For this review, take the finished solid that the model builds, in its own axes (mm). A direction names the side the tool comes from. Give positions to 0.01 mm unless a question says otherwise; leave off trailing zeros. Write each loop counter-clockwise with the first axis right and the second up, starting at its lowest first coordinate (ties: lowest second). Pieces come first, ordered by that corner, then holes.
Q1. We need section A-A (x = -74). Write out the cut boundary in (y, z), then the cut area to 3 significant figures.
Q2. We need section B-B (z = 41). Write out the cut boundary in (x, y), then the cut area to 3 significant figures.
Q3. Insertion check: P1, Ø1, axis at x = 100.5, z = 60, coming from the -Y side; P2, Ø1.4, axis at x = 12.5, y = 40.5, coming from the -Z side; P3, Ø5, axis at x = 157, z = 21.5, coming from the +Y side; P4, Ø5, axis at x = 86.5, y = 39, coming from the -Z side. Each pin has a flat end and moves straight along its axis. Give the tip position at first contact, or say it passes through.
Q4. Mouldability with a two-part tool opening along Y and no side actions: class faces 1 (the flat face through (2, 76, 10)), 2 (the flat face through (19.509, 47, 4)), 3 (the flat face through (4, 89.566, 7)), 4 (the cylindrical face through (4.839, 69.563, 4.056)) as released by +Y, released by -Y, zero draft, split by the parting line, or undercut.
Q5. For line 1 (X direction, y = 81.5, z = 18); line 2 (Z direction, x = 79, y = 84.5); line 3 (X direction, y = 51, z = 5.5), list the stretches that pass through material, from the lowest coordinate up.
Q6. We need section D-D (z = 20). Write out the cut boundary in (x, y).
Q7. We need section C-C (x = 161). Write out the cut boundary in (y, z).
Q8. Machinability: for faces 5 (the flat face through (-17.852, 25, 5)), 6 (the flat face through (-10.491, 47, 4)), 7 (the flat face through (4, 27, 10)), 8 (the flat face through (2, 74, 70)), 9 (the flat face through (26.87, 25, 5)), which of the approach directions +Z, -Z, +X, -X, +Y, -Y give a long, thin tool a straight path to every point of the face, cutting with its end or side? Answer none if there is none.
```python
from build123d import *

# Parameters (mm, degrees)
ESQUISSE2_W              = 430
ESQUISSE2_H              = 60
BOSS_EXTRU_1_DEPTH       = 80
ESQUISSE3_W              = 410
ESQUISSE3_H              = 60
ENL_V_MAT_EXTRU_2_DEPTH  = 50
BOSS_EXTRU_3_DEPTH       = 60
BOSS_EXTRU_4_DEPTH       = 20
ESQUISSE12_W             = 37.299463168
ESQUISSE12_H             = 2.901511437
ENL_V_MAT_EXTRU_3_DEPTH  = 80
ESQUISSE14_W             = 217.702790891
ESQUISSE14_H             = 66.731599488
ENL_V_MAT_EXTRU_4_DEPTH  = 80
ESQUISSE16_W             = 132.026208669
ESQUISSE16_H             = 23.789258621
ENL_V_MAT_EXTRU_5_DEPTH  = 80
ESQUISSE17_W             = 231.982221262
ESQUISSE17_H             = 63.124798286
ENL_V_MAT_EXTRU_6_DEPTH  = 80
ESQUISSE18_R             = 15
ENL_V_MAT_EXTRU_7_DEPTH  = 80
ENL_V_MAT_EXTRU_8_DEPTH  = 10
CONG_3_R                 = 2
CONG_4_R                 = 2
ESQUISSE26_W             = 44.72135955
ESQUISSE26_H             = 10
BOSS_EXTRU_5_DEPTH       = 10
ENL_V_MAT_EXTRU_9_DEPTH  = 10
ESQUISSE27_R             = 2
ENL_V_MAT_EXTRU_11_DEPTH = 10


with BuildPart() as part:
    # Esquisse2 → Boss.-Extru.1 (new body)
    with BuildSketch(Plane.XY):
        with Locations((4.509056244, 59.566253575)):
            Rectangle(ESQUISSE2_W, ESQUISSE2_H)
    extrude(amount=BOSS_EXTRU_1_DEPTH)

    # Esquisse3 → Enlèv. mat.-Extru.2 (cut)
    with BuildSketch(Plane(origin=(0, 89.566253575, 0), x_dir=(1, 0, 0), z_dir=(0, 1, 0))):
        with Locations((4.509056244, -40)):
            Rectangle(ESQUISSE3_W, ESQUISSE3_H)
    extrude(amount=-ENL_V_MAT_EXTRU_2_DEPTH, mode=Mode.SUBTRACT)

    # Esquisse5 → Boss.-Extru.3 (add)
    with BuildSketch(Plane.XY.offset(10)):
        Polygon((-200.490943756, 59.566253575), (-200.490943756, 39.566253575), (4.509056244, 39.566253575), align=None)
        Polygon((209.509056244, 59.566253575), (4.509056244, 39.566253575), (209.509056244, 39.566253575), align=None)
    extrude(amount=BOSS_EXTRU_3_DEPTH)

    # Esquisse11 → Boss.-Extru.4 (add)
    with BuildSketch(Plane(origin=(3.732634391, 37.450765056, -5.350109294), x_dir=(0.995167757, -0.097202432, 0.013886062), z_dir=(0.098189284, 0.985165817, -0.140737974))):
        Polygon((0.78019193, -15.495008178), (-209.853755734, -12.986939636), (-207.594167279, -81.787183383), (2.874639564, -83.936671883), align=None)
    boss_extru_4 = extrude(amount=-BOSS_EXTRU_4_DEPTH)

    # Esquisse12 → Enlèv. mat.-Extru.3 (cut)
    with BuildSketch(Plane(origin=(0, 89.566253575, 0), x_dir=(1, 0, 0), z_dir=(0, 1, 0))):
        with Locations((-6.67152918, -81.450755719)):
            Rectangle(ESQUISSE12_W, ESQUISSE12_H)
    extrude(amount=-ENL_V_MAT_EXTRU_3_DEPTH, mode=Mode.SUBTRACT)

    # Esquisse14 → Enlèv. mat.-Extru.4 (cut)
    with BuildSketch(Plane.XY.offset(80)):
        with Locations((-32.350917278, -3.799546169)):
            Rectangle(ESQUISSE14_W, ESQUISSE14_H)
    extrude(amount=-ENL_V_MAT_EXTRU_4_DEPTH, mode=Mode.SUBTRACT)

    # Symétrie3: Boss.-Extru.4 across plane
    add(boss_extru_4.mirror(Plane(origin=(4.509056244, 0, 0), x_dir=(0, 0, 1), z_dir=(1, 0, 0))))

    # Esquisse16 → Enlèv. mat.-Extru.5 (cut)
    with BuildSketch(Plane(origin=(0, 89.566253575, 0), x_dir=(1, 0, 0), z_dir=(0, 1, 0))):
        with Locations((17.978222552, -91.89462931)):
            Rectangle(ESQUISSE16_W, ESQUISSE16_H)
    extrude(amount=-ENL_V_MAT_EXTRU_5_DEPTH, mode=Mode.SUBTRACT)

    # Esquisse17 → Enlèv. mat.-Extru.6 (cut)
    with BuildSketch(Plane.XY.offset(80)):
        with Locations((69.126673961, -1.996145568)):
            Rectangle(ESQUISSE17_W, ESQUISSE17_H)
    extrude(amount=-ENL_V_MAT_EXTRU_6_DEPTH, mode=Mode.SUBTRACT)

    # Esquisse18 → Enlèv. mat.-Extru.7 (cut)
    with BuildSketch(Plane.XY.offset(10)):
        with Locations((4.509056244, 54.566253575)):
            Circle(ESQUISSE18_R)
    extrude(amount=-ENL_V_MAT_EXTRU_7_DEPTH, mode=Mode.SUBTRACT)

    # Esquisse20 → Enlèv. mat.-Extru.8 (cut)
    with BuildSketch(Plane(origin=(0, 0, 0), x_dir=(-1, 0, 0), z_dir=(0, 0, -1))):
        Polygon((-19.509056244, 54.566253575), (-19.509056244, 39.566253575), (-4.509056244, 39.566253575), (10.490943756, 39.566253575), (10.490943756, 54.566253575), align=None)
    extrude(amount=-ENL_V_MAT_EXTRU_8_DEPTH, mode=Mode.SUBTRACT)

    # Congé3
    cong_3_edges = [part.edges().sort_by_distance(p)[0] for p in [
        (4.509056244, 69.566253575, 10),
        (-10.490943756, 47.81376188, 10),
        (19.509056244, 47.81376188, 10),
    ]]
    fillet(cong_3_edges, radius=CONG_3_R)

    # Congé4
    cong_4_edges = [part.edges().sort_by_distance(p)[0] for p in [
        (19.509056244, 40.31376188, 10),
        (-10.490943756, 40.31376188, 10),
    ]]
    fillet(cong_4_edges, radius=CONG_4_R)

    # Esquisse26 → Boss.-Extru.5 (add)
    with BuildSketch(Plane.XZ.offset(-29.566253575)):
        with Locations((4.509056244, 5)):
            Rectangle(ESQUISSE26_W, ESQUISSE26_H)
    extrude(amount=BOSS_EXTRU_5_DEPTH)

    # Esquisse24 → Enlèv. mat.-Extru.9 (cut)
    with BuildSketch(Plane(origin=(0, 0, 0), x_dir=(-1, 0, 0), z_dir=(0, 0, -1))):
        with BuildLine():
            ThreePointArc((-2.510656885, 24.646253575), (-4.509056244, 26.566253575), (-6.507455604, 24.646253575))
            ThreePointArc((-6.507455604, 24.646253575), (-4.509056244, 24.566253575), (-2.510656885, 24.646253575))
        make_face()
        with BuildLine():
            ThreePointArc((-2.510656885, 24.646253575), (-4.509056244, 24.566253575), (-6.507455604, 24.646253575))
            ThreePointArc((-6.507455604, 24.646253575), (-4.54906425, 22.566653775), (-2.509056244, 24.566253575))
            ThreePointArc((-2.509056244, 24.566253575), (-2.509456444, 24.60626158), (-2.510656885, 24.646253575))
        make_face()
    extrude(amount=-ENL_V_MAT_EXTRU_9_DEPTH, mode=Mode.SUBTRACT)

    # Esquisse27 → Enlèv. mat.-Extru.11 (cut)
    with BuildSketch(Plane(origin=(0, 0, 0), x_dir=(-1, 0, 0), z_dir=(0, 0, -1))):
        with Locations((-4.509056244, 82.566253575)):
            Circle(ESQUISSE27_R)
    extrude(amount=-ENL_V_MAT_EXTRU_11_DEPTH, mode=Mode.SUBTRACT)


solid = part.part
```
Computed:
1. outline: (29.57, 0) - (89.57, 0) - (89.57, 10) - (47.39, 10) - (55.96, 70) - (89.57, 70) - (89.57, 80) - (29.57, 80) - close
1. area: 2,530 mm2
2. outline: (-210.49, 29.57) - (219.51, 29.57) - (219.51, 89.57) - (209.51, 89.57) - (209.51, 64.43) - (4.51, 43.99) - (-200.49, 64.43) - (-200.49, 89.57) - (-210.49, 89.57) - close
2. area: 11,300 mm2
3. P1: stops at y = 29.57
3. P2: stops at z = 10
3. P3: stops at y = 56.84
3. P4: stops at z = 0
4. face 1: zero draft
4. face 2: undercut
4. face 3: released by +Y
4. face 4: undercut
5. line 1: x = -210.49 to -200.49, 209.51 to 219.51
5. line 2: z = 0 to 10, 70 to 80
5. line 3: x = -210.49 to -10.49, 19.51 to 219.51
6. outline: (-210.49, 29.57) - (219.51, 29.57) - (219.51, 89.57) - (209.51, 89.57) - (209.51, 61.43) - (4.51, 40.99) - (-200.49, 61.43) - (-200.49, 89.57) - (-210.49, 89.57) - close
7. outline: (29.57, 0) - (89.57, 0) - (89.57, 10) - (55.16, 10) - (63.73, 70) - (89.57, 70) - (89.57, 80) - (29.57, 80) - close
8. face 5: +Z, -Z, -X, -Y
8. face 6: -Z
8. face 7: +Z, +X, -X, -Y
8. face 8: +Y
8. face 9: +Z, -Z, +X, -Y
